Verification items for the finished model (mm, model axes). Face numbers are marked on the shaded views. Round coordinates to 2 decimals unless told otherwise and drop trailing zeros. Order: outer loops, then holes, each group sorted by start corner. A loop starts at its lowest first (then second) coordinate and runs counter-clockwise, first axis right, second up.
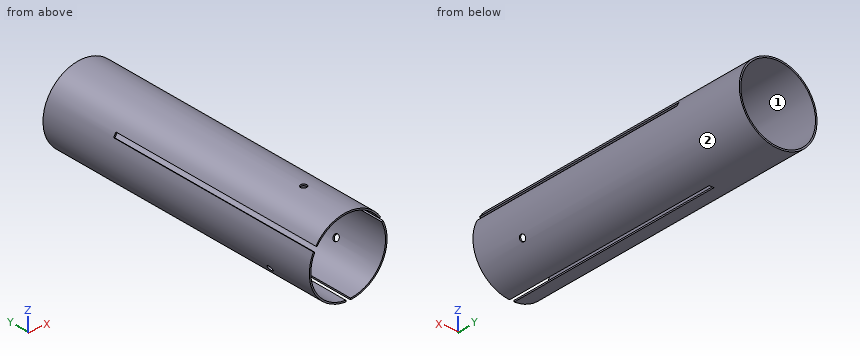
```python
from build123d import *

# Parameters (mm, degrees)
SKETCH2_R           = 39.624
SKETCH2_R_2         = 38.1
BOSS_EXTRUDE1_DEPTH = 304.8
SKETCH3_W           = 4.7625
SKETCH3_H           = 228.6
CUT_EXTRUDE1_DEPTH  = 310.908313461
CIRPATTERN1_COUNT   = 3
SKETCH4_R           = 3.175
CUT_EXTRUDE3_DEPTH  = 310.908313461
CIRPATTERN2_COUNT   = 3


with BuildPart() as part:
    # Sketch2 → Boss-Extrude1 (new body)
    with BuildSketch(Plane(origin=(0, 0, 0), x_dir=(1, 0, 0), z_dir=(0, 1, 0))):
        with Locations(Location((0, 0, 0), (0, 0, 90))):
            Circle(SKETCH2_R)
        with Locations(Location((0, 0, 0), (0, 0, 90))):
            Circle(SKETCH2_R_2, mode=Mode.SUBTRACT)
    extrude(amount=BOSS_EXTRUDE1_DEPTH)

    # Sketch3 → Cut-Extrude1 (cut, through all)
    with BuildSketch(Plane.XY):
        with Locations((0, 114.3)):
            Rectangle(SKETCH3_W, SKETCH3_H)
    cut_extrude1 = extrude(amount=-CUT_EXTRUDE1_DEPTH, mode=Mode.SUBTRACT)

    # CirPattern1: Cut-Extrude1 ×3 about axis
    cirpattern1_axis = Axis((0, 0, 0), (0, 1, 0))
    for i in range(1, CIRPATTERN1_COUNT):
        add(cut_extrude1.rotate(cirpattern1_axis, i * 360 / CIRPATTERN1_COUNT), mode=Mode.SUBTRACT)

    # Sketch4 → Cut-Extrude3 (cut, through all)
    with BuildSketch(Plane.XY):
        with Locations(Location((0, 50.8, 0), (0, 0, 180))):
            Circle(SKETCH4_R)
    cut_extrude3 = extrude(amount=CUT_EXTRUDE3_DEPTH, mode=Mode.SUBTRACT)

    # CirPattern2: Cut-Extrude3 ×3 about axis
    cirpattern2_axis = Axis((0, 304.8, 0), (0, -1, 0))
    for i in range(1, CIRPATTERN2_COUNT):
        add(cut_extrude3.rotate(cirpattern2_axis, i * 360 / CIRPATTERN2_COUNT), mode=Mode.SUBTRACT)


solid = part.part
```
1) Sectioned sample at C-C on z = 0. Record the cut outline in (x, y), then the cut area to 3 significant figures.
2) Sectioned sample at A-A on y = 111. Record the cut outline in (x, z), then the cut area to 3 significant figures.
3) Draft check along Z on the marked faces 1 and 2. Enter one of: released by +Z, released by -Z, zero draft, split by the parting line, or undercut.
4) Scan lines: probe 1 along Y at (x, z) = (0, 38.8) (3 decimals); probe 2 along Z at (x, y) = (0, 73); probe 3 along Z at (x, y) = (18, 120.5). Record each from-to range of solid material in increasing order.
5) Sectioned sample at B-B on x = 22. Record the cut outline in (y, z).
6) Go/stop test with flat-tipped pins: pin 1 Ø4 at (x, z) = (34, 20) entering from -Y; pin 2 Ø6 at (x, y) = (2, 201) entering from -Z; pin 3 Ø4 at (x, y) = (21, 218.5) entering from +Z. Record where each tip stops, or that it passes through.
7) Sectioned sample at D-D on y = 256. Record the cut outline in (x, z), then the cut area to 3 significant figures.
Returned:
1. outline: (-39.62, 0) - (-38.1, 0) - (-38.1, 304.8) - (-39.62, 304.8) - close; (38.1, 0) - (39.62, 0) - (39.62, 304.8) - (38.1, 304.8) - close
1. area: 929 mm2
2. outline: (-35.44, 17.71) arc R39.62 ccw to (-2.38, -39.55) - (-2.38, -38.03) arc R38.1 cw to (-34.12, 16.95) - close; (-33.06, 21.84) - (-31.74, 21.07) arc R38.1 cw to (31.74, 21.07) - (33.06, 21.84) arc R39.62 ccw to start; (2.38, -39.55) arc R39.62 ccw to (35.44, 17.71) - (34.12, 16.95) arc R38.1 cw to (2.38, -38.03) - close
2. area: 350 mm2
3. face 1: undercut
3. face 2: split by the parting line
4. probe 1: y = 0 to 47.625, 53.975 to 304.8
4. probe 2: z = 38.1 to 39.62
4. probe 3: z = -35.3 to -33.58, 33.58 to 35.3
5. outline: (0, -32.96) - (304.8, -32.96) - (304.8, -31.11) - (0, -31.11) - close; (0, 31.11) - (304.8, 31.11) - (304.8, 32.96) - (0, 32.96) - close
6. pin 1: stops at y = 228.6
6. pin 2: stops at z = -39.55
6. pin 3: stops at z = 34.77
7. outline: circle Ø79.25 at (0, 0); hole circle Ø76.2 at (0, 0)
7. area: 372 mm2
